Autodesk Fusion 360 part; units mm, degrees
sketch "Esquisse1" plane through (0, 0, 0) normal (0, 0, 1) x (1, 0, 0)
  line L0 (21.0537, 17.2704) -> (26.0537, 17.2704)
  line L1 (26.0537, 17.2704) -> (26.0537, 15.2704)
  line L2 (26.0537, 15.2704) -> (21.0537, 15.2704)
  line L3 (21.0537, 15.2704) -> (21.0537, 17.2704)
  dimension "d1" = 5
  dimension "d2" = 2
extrude "Extrusion1" add sketch "Esquisse1" along normal blind 6
sketch "Esquisse2" plane through (0, 17.2704, 0) normal (0, 1, 0) x (-1, 0, 0)
  line L0 (-26.0537, 0) -> (-21.0537, 0)
  line L1 (-21.0537, 0) -> (-21.0537, 6)
  line L2 (-21.0537, 6) -> (-26.0537, 6)
  line L3 (-26.0537, 6) -> (-26.0537, 0)
  line L4 (-21.0537, 6) -> (-26.0537, 6)
  line L5 (-26.0537, 6) -> (-26.0537, 4.1)
  line L6 (-26.0537, 4.1) -> (-21.0537, 4.1)
  line L7 (-21.0537, 4.1) -> (-21.0537, 6)
  dimension "d5" = 1.9
extrude "Extrusion2" add sketch "Esquisse2" along normal blind 1.9 contours L1 L2 L3 L4 L5 L6 L7
Design review of the part built by this model. Coordinates are the model's own, in mm. A direction names the side the tool comes from. Coordinates: 2 decimals unless noted, no trailing zeros. Order: outer loops, then holes, each group sorted by start corner. A loop starts at its lowest first (then second) coordinate and runs counter-clockwise, first axis right, second up. Notation, with made-up numbers: (-35.75, 64.5) -> (-6.75, 64.5) arc R8 cw to (-6.75, 76.5) -> close; hole circle Ø6 at (0, 84.25). An arc over 180 degrees is marked (long way). One line per item, written item: value. Start each with the question number.
Q1. Take a section at C-C, the plane z = 2.8. State the section outline as (x, y) points, then the cut area to 4 significant figures.
Q2. For probe 1 along Y at (x, z) = (23.95, 3.55); probe 2 along Z at (x, y) = (21.75, 17.75), list the stretches that pass through material, from the lowest coordinate up.
Q3. Tool access review of faces 1 (the flat face through (24, 15.27, 3)), 2 (the flat face through (24, 18, 4.1)): name each direction out of +Z, -Z, +X, -X, +Y, -Y from which nothing blocks a thin tool from reaching the whole face with its end or side.
Q4. Take a section at A-A, the plane x = 25.25. State the section outline as (y, z) points, then the cut area to 3 significant figures.
Q5. Insertion check: pin 1 Ø0.6 at (x, y) = (24.5, 18) entering from -Z; pin 2 Ø1.5 at (x, z) = (23, 2) entering from +Y. Each pin has a flat end and moves straight along its axis. Give the tip position at first contact, or say it passes through.
Q6. Take a section at B-B, the plane y = 18.7. State the section outline as (x, z) points, then the cut area to 3 significant figures.
Values follow:
1. outline: (21.05, 15.27) -> (26.05, 15.27) -> (26.05, 17.27) -> (21.05, 17.27) -> close
1. area: 10.00 mm2
2. probe 1: y = 15.27 to 17.27
2. probe 2: z = 4.1 to 6
3. face 1: +Z, -Z, +X, -X, -Y
3. face 2: -Z, +X, -X, +Y
4. outline: (15.27, 0) -> (17.27, 0) -> (17.27, 4.1) -> (19.17, 4.1) -> (19.17, 6) -> (15.27, 6) -> close
4. area: 15.6 mm2
5. pin 1: stops at z = 4.1
5. pin 2: stops at y = 17.27
6. outline: (21.05, 4.1) -> (26.05, 4.1) -> (26.05, 6) -> (21.05, 6) -> close
6. area: 9.50 mm2
